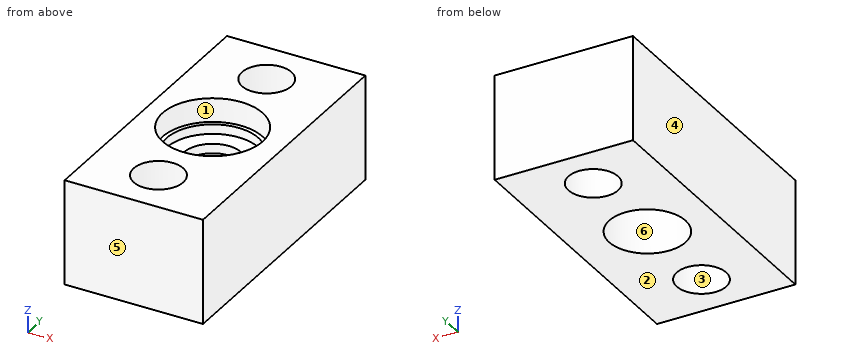
```python
from build123d import *

# Parameters (mm, degrees)
SKETCH1_W               = 15
SKETCH1_H               = 30
BOSS_EXTRUDE1_DEPTH     = 6
SKETCH2_R               = 5.25
CUT_EXTRUDE1_DEPTH      = 2.5
SKETCH4_R               = 4.8
CUT_EXTRUDE3_DEPTH      = 1
SKETCH5_R               = 2.36
CUT_EXTRUDE4_DEPTH      = 4.5
CUT_EXTRUDE4_DEPTH_BACK = 5
CUT_EXTRUDE6_DEPTH      = 7
CUT_EXTRUDE6_DEPTH_BACK = 1
SKETCH11_W              = 14.5
SKETCH11_H              = 30
BOSS_EXTRUDE5_DEPTH     = 5
SKETCH12_R              = 4
CUT_EXTRUDE8_DEPTH      = 5
SKETCH13_R              = 2.595
CUT_EXTRUDE9_DEPTH      = 12
SKETCH14_R              = 3
CUT_EXTRUDE10_DEPTH     = 1


with BuildPart() as part:
    # Sketch1 → Boss-Extrude1 (new body)
    with BuildSketch(Plane.XY):
        Rectangle(SKETCH1_W, SKETCH1_H)
    extrude(amount=BOSS_EXTRUDE1_DEPTH)

    # Sketch2 → Cut-Extrude1 (cut)
    with BuildSketch(Plane.XY.offset(6)):
        Circle(SKETCH2_R)
    extrude(amount=-CUT_EXTRUDE1_DEPTH, mode=Mode.SUBTRACT)

    # Sketch4 → Cut-Extrude3 (cut)
    with BuildSketch(Plane.XY.offset(3.5)):
        Circle(SKETCH4_R)
    extrude(amount=-CUT_EXTRUDE3_DEPTH, mode=Mode.SUBTRACT)

    # Sketch5 → Cut-Extrude4 (cut, two sides)
    with BuildSketch(Plane.XY.offset(2.5)) as cut_extrude4_sk:
        Circle(SKETCH5_R)
    extrude(amount=CUT_EXTRUDE4_DEPTH, mode=Mode.SUBTRACT)
    extrude(cut_extrude4_sk.sketch, amount=-CUT_EXTRUDE4_DEPTH_BACK, mode=Mode.SUBTRACT)

    # Sketch6 → Cut-Extrude6 (cut, two sides)
    with BuildSketch(Plane.XY) as cut_extrude6_sk:
        Polygon((-7, 91.640828326), (-7, 15), (-7, -15), (-7, -91.640828326), (-160.281656652, -91.640828326), (-160.281656652, 91.640828326), align=None)
    extrude(amount=CUT_EXTRUDE6_DEPTH, mode=Mode.SUBTRACT)
    extrude(cut_extrude6_sk.sketch, amount=-CUT_EXTRUDE6_DEPTH_BACK, mode=Mode.SUBTRACT)

    # Sketch11 → Boss-Extrude5 (add)
    with BuildSketch(Plane(origin=(0, 0, 0), x_dir=(-1, 0, 0), z_dir=(0, 0, -1))):
        with Locations((-0.25, 0)):
            Rectangle(SKETCH11_W, SKETCH11_H)
    extrude(amount=BOSS_EXTRUDE5_DEPTH)

    # Sketch12 → Cut-Extrude8 (cut)
    with BuildSketch(Plane(origin=(0, 0, -5), x_dir=(-1, 0, 0), z_dir=(0, 0, -1))):
        Circle(SKETCH12_R)
    extrude(amount=-CUT_EXTRUDE8_DEPTH, mode=Mode.SUBTRACT)

    # Sketch13 → Cut-Extrude9 (cut, through all)
    with BuildSketch(Plane(origin=(0, 0, -5), x_dir=(-1, 0, 0), z_dir=(0, 0, -1))):
        with Locations((0, -10)):
            Circle(SKETCH13_R)
        with Locations((0, 10)):
            Circle(SKETCH13_R)
    extrude(amount=-CUT_EXTRUDE9_DEPTH, mode=Mode.SUBTRACT)

    # Sketch14 → Cut-Extrude10 (cut)
    with BuildSketch(Plane.XY.offset(2.5)):
        Circle(SKETCH14_R)
    extrude(amount=-CUT_EXTRUDE10_DEPTH, mode=Mode.SUBTRACT)


solid = part.part
```
Input: part model. Units: mm. Frame: model coordinates. Face numbers are marked on the shaded views. A direction names the side the tool comes from. Round coordinates to 2 decimals unless told otherwise and drop trailing zeros. Loops run counter-clockwise (first coordinate to the right, second up) from the corner with the lowest first, then second, coordinate; pieces in that order, holes last. Notation, with made-up numbers: (77.5, 14.25) -> (125.5, 14.25) arc R10 cw to (125.5, 33.25) -> close; hole circle Ø6 at (28.5, -5.75). An arc over 180 degrees is marked (long way). One line per item, written item: value.
(1) Set-up query: the marked faces 1 and 2. Return all of +Z, -Z, +X, -X, +Y, -Y with unobstructed straight access to the full face (end or side cutting, diameter ignored); none if empty.
Geometry check:
face 1: +Z
face 2: -Z, +X, -X, +Y, -Y
(2) Section D-D (y = 0). Return the cut outline in (x, z).
Geometry check:
outline: (-7, -5) -> (-4, -5) -> (-4, 0) -> (-2.36, 0) -> (-2.36, 1.5) -> (-3, 1.5) -> (-3, 2.5) -> (-4.8, 2.5) -> (-4.8, 3.5) -> (-5.25, 3.5) -> (-5.25, 6) -> (-7, 6) -> close; (2.36, 0) -> (4, 0) -> (4, -5) -> (7.5, -5) -> (7.5, 6) -> (5.25, 6) -> (5.25, 3.5) -> (4.8, 3.5) -> (4.8, 2.5) -> (3, 2.5) -> (3, 1.5) -> (2.36, 1.5) -> close
(3) Material intervals for line 1 (Y direction, x = 0, z = -2.35) (3 decimals); line 2 (Y direction, x = 0, z = 2.35) (3 decimals); line 3 (X direction, y = 8.75, z = -2), sorted ascending. Write a range as [from, to].
Geometry check:
line 1: [-15, -12.595], [-7.405, -4], [4, 7.405], [12.595, 15]
line 2: [-15, -12.595], [-7.405, -3], [3, 7.405], [12.595, 15]
line 3: [-7, -2.27], [2.27, 7.5]
(4) Pin query (flat end, axial travel): pin 1 (7 mm diameter, centred on x = 0, y = 0, fed in from +Z); pin 2 (7.5 mm diameter, centred on x = 0, y = 0, fed in from -Z); pin 3 (5 mm diameter, centred on x = 0, y = -2.5, fed in from +Z). Return the tip coordinate at first contact, or that it passes through.
Geometry check:
pin 1: z = 2.5
pin 2: z = 0
pin 3: z = 3.5
(5) Mould query, pull axis Y, two halves, no side actions, for the marked faces 3, 4, 5 and 6. Classes: pulls with the +Y half, pulls with the -Y half, needs draft (parallel to the pull), parting line crosses it, or undercut.
Geometry check:
face 3: undercut
face 4: needs draft
face 5: pulls with the -Y half
face 6: undercut
(6) Section C-C (z = -4). Return the cut outline in (x, y) (3 decimals).
Geometry check:
outline: (-7, -15) -> (7.5, -15) -> (7.5, 15) -> (-7, 15) -> close; hole circle Ø8 at (0, 0); hole circle Ø5.19 at (0, -10); hole circle Ø5.19 at (0, 10)
(7) Section B-B (x = 0). Give the number of separate pieces and of enclosed holes in the cut face, plus the area to 3 significant figures.
Geometry check:
separate pieces: 4
enclosed holes: 0
area: 127 mm2
(8) Section A-A (y = 10). Return the cut outline in (x, z) (3 decimals), plus the area to 3 significant figures.
Geometry check:
outline: (-7, -5) -> (-2.595, -5) -> (-2.595, 6) -> (-7, 6) -> close; (2.595, -5) -> (7.5, -5) -> (7.5, 6) -> (2.595, 6) -> close
area: 102 mm2
